from build123d import *

# Parameters (mm, degrees)
SKETCH1_R           = 71.8312
SKETCH1_R_2         = 9.525
BOSS_EXTRUDE1_DEPTH = 6.35
CUT_EXTRUDE1_START  = -6.35
CUT_EXTRUDE1_DEPTH  = 6.35
CIRPATTERN1_COUNT   = 4


# Read off the part's stored shape, not the designer's step: Cut-Extrude1
with BuildPart() as part:
    # Sketch1 → Boss-Extrude1 (new body)
    with BuildSketch(Plane(origin=(0, 0, 0), x_dir=(1, 0, 0), z_dir=(0, 1, 0))):
        with Locations(Location((0, 0, 0), (0, 0, 270))):
            Circle(SKETCH1_R)
        with Locations(Location((0, 0, 0), (0, 0, 270))):
            Circle(SKETCH1_R_2, mode=Mode.SUBTRACT)
    extrude(amount=BOSS_EXTRUDE1_DEPTH)

    # Cut-Extrude1 outline → Cut-Extrude1 (cut)
    with BuildSketch(Plane(origin=(0, 6.35, 0), x_dir=(1, 0, 0), z_dir=(0, 1, 0)).offset(CUT_EXTRUDE1_START)):
        with BuildLine():
            ThreePointArc((-12.751963692, -23.169060792), (-12.751963692, -12.751963692), (-23.169060792, -12.751963692))
            Line((-23.169060792, -12.751963692), (-55.733113553, -45.316016453))
            ThreePointArc((-55.733113553, -45.316016453), (-50.792328621, -50.792328621), (-45.316016453, -55.733113553))
            Line((-45.316016453, -55.733113553), (-12.751963692, -23.169060792))
        make_face()
        with BuildLine():
            ThreePointArc((-66.4688917, 27.232475642), (-71.8312, 0), (-66.4688917, -27.232475642))
            ThreePointArc((-66.4688917, -27.232475642), (-57.15, 0), (-66.4688917, 27.232475642))
        make_face()
    cut_extrude1 = extrude(amount=CUT_EXTRUDE1_DEPTH, mode=Mode.SUBTRACT)

    # CirPattern1: Cut-Extrude1 ×4 about axis
    cirpattern1_axis = Axis((0, 0, 0), (0, 1, 0))
    for i in range(1, CIRPATTERN1_COUNT):
        add(cut_extrude1.rotate(cirpattern1_axis, i * 360 / CIRPATTERN1_COUNT), mode=Mode.SUBTRACT)


solid = part.part
Work out the finished part from the listing and answer in its coordinate system (mm). A direction names the side the tool comes from. Give positions to 0.01 mm unless a question says otherwise; leave off trailing zeros. Write each loop counter-clockwise with the first axis right and the second up, starting at its lowest first coordinate (ties: lowest second). Pieces come first, ordered by that corner, then holes. Notation, with made-up numbers: M 74,-20 L 111,-20 A25 cw 111,6 Z; hole C 18,16 d1. An arc over 180 degrees is marked long. Answer as CSV lines item,"result".
Q1. The mould has two halves that part along Z. Classify faces 1 (the cylindrical face through (36.8, 3.13, -61.69)), 2 (the cylindrical face through (-12.639, 3.131, 12.868)), 3 (the cylindrical face through (-61.842, 3.131, 36.542)): +Z half, -Z half, draft (parallel to the pull), parting line (faces both ways), or undercut.
A:
face 1,"-Z half"
face 2,"undercut"
face 3,"+Z half"
Q2. Given P1, Ø8, axis at x = 21, z = -19, coming from the -Y side; P2, Ø1, axis at y = 0.5, z = 18.5, coming from the +X side; P3, Ø1.5, axis at y = 5.5, z = -16, coming from the +X side; P4, Ø1, axis at y = 1, z = -34, coming from the -X side, each flat-ended and moving along its own axis, determine where each tip first touches the part or whether it passes through.
A:
P1,"passes through"
P2,"stops at x = 61.42"
P3,"stops at x = 60.43"
P4,"stops at x = -63.54"
Q3. Find the intervals of material crossed by probe 1 along X at (y, z) = (4.25, 29.5); probe 2 along X at (y, z) = (3, 40.5); probe 3 along Z at (x, y) = (-33.5, 3.25), in increasing order. Write a range as [from, to].
A:
probe 1,"x = [-65.49, -39.92], [-19.08, 19.08], [39.92, 65.49]"
probe 2,"x = [-59.33, -50.92], [-30.08, 30.08], [50.92, 59.33]"
probe 3,"z = [-63.54, -43.92], [-23.08, 23.08], [43.92, 63.54]"
Q4. A cutting plane is placed at C-C on z = 0. Write down the section's boundary in (x, y) (3 decimals).
A:
outline,"M -57.15,0 L -9.525,0 L -9.525,6.35 L -57.15,6.35 Z; M 9.525,0 L 57.15,0 L 57.15,6.35 L 9.525,6.35 Z"
Q5. A cutting plane is placed at B-B on x = 0. Write down the section's boundary in (y, z) (3 decimals).
A:
outline,"M 0,-57.15 L 6.35,-57.15 L 6.35,-9.525 L 0,-9.525 Z; M 0,9.525 L 6.35,9.525 L 6.35,57.15 L 0,57.15 Z"
Q6. A cutting plane is placed at A-A on y = 2.5. Write down the section's boundary in (x, z) (3 decimals).
A:
outline,"M -66.469,-27.232 A71.831 ccw -55.733,-45.316 L -23.169,-12.752 A7.366 cw -12.752,-23.169 L -45.316,-55.733 A71.831 ccw -27.232,-66.469 A44.45 cw 27.232,-66.469 A71.831 ccw 45.316,-55.733 L 12.752,-23.169 A7.366 cw 23.169,-12.752 L 55.733,-45.316 A71.831 ccw 66.469,-27.232 A44.45 cw 66.469,27.232 A71.831 ccw 55.733,45.316 L 23.169,12.752 A7.366 cw 12.752,23.169 L 45.316,55.733 A71.831 ccw 27.232,66.469 A44.45 cw -27.232,66.469 A71.831 ccw -45.316,55.733 L -12.752,23.169 A7.366 cw -23.169,12.752 L -55.733,45.316 A71.831 ccw -66.469,27.232 A44.45 cw Z; hole C 0,0 d19.05"
Q7. A cutting plane is placed at D-D on z = 16. Write down the section's boundary in (x, y).
A:
outline,"M -60.13,0 L -26.42,0 L -26.42,6.35 L -60.13,6.35 Z; M -10.86,0 L 10.86,0 L 10.86,6.35 L -10.86,6.35 Z; M 26.42,0 L 60.13,0 L 60.13,6.35 L 26.42,6.35 Z"
Q8. A tool of negligible diameter and unlimited length cuts with its end or side. For faces 4 (the flat face through (-39.679, 3.131, -29.262)), 5 (the cylindrical face through (-57.15, 3.13, 0.41)), from which of +Z, -Z, +X, -X, +Y, -Y can it reach the whole face along a straight path? Write none if from no direction.
A:
face 4,"+Y, -Y"
face 5,"-X, +Y, -Y"
